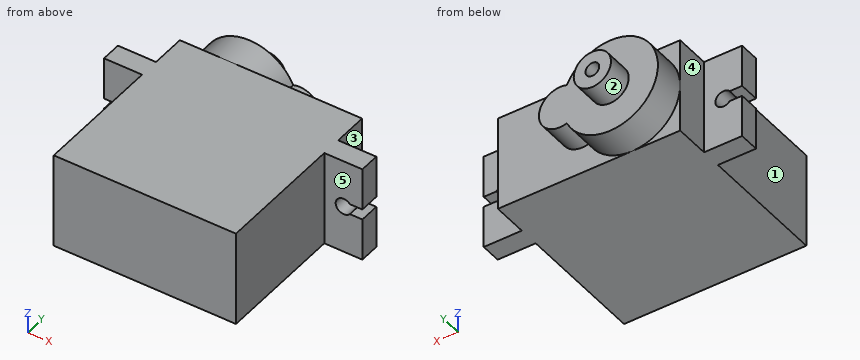
```python
from build123d import *

# Parameters (mm, degrees)
ESBO_O1_W                  = 22.5
ESBO_O1_H                  = 11.8
RESSALTO_EXTRUS_O1_DEPTH   = 22.7
ESBO_O2_W                  = 11.8
ESBO_O2_H                  = 2.5
RESSALTO_EXTRUS_O2_DEPTH   = 4.7
RESSALTO_EXTRUS_O3_DEPTH   = 4.7
RESSALTO_EXTRUS_O4_DEPTH   = 4
ESBO_O5_R                  = 2.3
ESBO_O5_R_2                = 0.85
RESSALTO_EXTRUS_O5_DEPTH   = 3.2
CORTE_EXTRUS_O1_DEPTH      = 35.894698738
CORTE_EXTRUS_O1_DEPTH_BACK = 3.2
CORTE_EXTRUS_O2_DEPTH      = 35.894698738
CORTE_EXTRUS_O2_DEPTH_BACK = 3.2


with BuildPart() as part:
    # Esboço1 → Ressalto-extrusão1 (new body)
    with BuildSketch(Plane(origin=(0, 0, 0), x_dir=(1, 0, 0), z_dir=(0, 1, 0))):
        with Locations((11.25, 5.9)):
            Rectangle(ESBO_O1_W, ESBO_O1_H)
    extrude(amount=RESSALTO_EXTRUS_O1_DEPTH)

    # Esboço2 → Ressalto-extrusão2 (add)
    with BuildSketch(Plane.ZY):
        with Locations((-5.9, 17.15)):
            Rectangle(ESBO_O2_W, ESBO_O2_H)
    extrude(amount=RESSALTO_EXTRUS_O2_DEPTH)

    # Esboço3 → Ressalto-extrusão3 (add)
    with BuildSketch(Plane(origin=(22.5, 0, 0), x_dir=(0, 0, -1), z_dir=(1, 0, 0))):
        Polygon((5.9, 15.9), (11.8, 15.9), (11.8, 18.4), (0, 18.4), (0, 15.9), align=None)
    extrude(amount=RESSALTO_EXTRUS_O3_DEPTH)

    # Esboço4 → Ressalto-extrusão4 (add)
    with BuildSketch(Plane(origin=(0, 22.7, 0), x_dir=(1, 0, 0), z_dir=(0, 1, 0))):
        with BuildLine():
            ThreePointArc((11.244155686, 8.4), (0, 5.9), (11.244155686, 3.4))
            ThreePointArc((11.244155686, 3.4), (14.7, 5.9), (11.244155686, 8.4))
        make_face()
    extrude(amount=RESSALTO_EXTRUS_O4_DEPTH)

    # Esboço5 → Ressalto-extrusão5 (add)
    with BuildSketch(Plane(origin=(0, 26.7, 0), x_dir=(1, 0, 0), z_dir=(0, 1, 0))):
        with Locations(Location((5.9, 5.9, 0), (0, 0, 90))):
            Circle(ESBO_O5_R)
        with Locations(Location((5.9, 5.9, 0), (0, 0, 270))):
            Circle(ESBO_O5_R_2, mode=Mode.SUBTRACT)
    extrude(amount=RESSALTO_EXTRUS_O5_DEPTH)

    # Esboço6 → Corte-extrusão1 (cut, two sides: drawn at the far end of the back side and taken through both)
    with BuildSketch(Plane(origin=(0, 18.4, 0), x_dir=(1, 0, 0), z_dir=(0, 1, 0)).offset(-CORTE_EXTRUS_O1_DEPTH_BACK)):
        with BuildLine():
            Line((-3.159934208, 6.55), (-4.7, 6.55))
            Line((-4.7, 6.55), (-4.7, 5.25))
            Line((-4.7, 5.25), (-3.159934208, 5.25))
            ThreePointArc((-3.159934208, 5.25), (-1.4, 5.9), (-3.159934208, 6.55))
        make_face()
    extrude(amount=CORTE_EXTRUS_O1_DEPTH + CORTE_EXTRUS_O1_DEPTH_BACK, mode=Mode.SUBTRACT)

    # Esboço7 → Corte-extrusão2 (cut, two sides: drawn at the far end of the back side and taken through both)
    with BuildSketch(Plane(origin=(0, 18.4, 0), x_dir=(1, 0, 0), z_dir=(0, 1, 0)).offset(-CORTE_EXTRUS_O2_DEPTH_BACK)):
        with BuildLine():
            Line((25.659934208, 5.25), (27.2, 5.25))
            Line((27.2, 5.25), (27.2, 6.55))
            Line((27.2, 6.55), (25.659934208, 6.55))
            ThreePointArc((25.659934208, 6.55), (23.9, 5.9), (25.659934208, 5.25))
        make_face()
    extrude(amount=CORTE_EXTRUS_O2_DEPTH + CORTE_EXTRUS_O2_DEPTH_BACK, mode=Mode.SUBTRACT)


solid = part.part
```
Work out the finished part from the listing and answer in its coordinate system (mm). Face numbers are marked on the shaded views. A direction names the side the tool comes from. Coordinates: 2 decimals unless noted, no trailing zeros. Order: outer loops, then holes, each group sorted by start corner. A loop starts at its lowest first (then second) coordinate and runs counter-clockwise, first axis right, second up. Notation, with made-up numbers: M 69,-13 L 74,-13 A25 ccw 74,15 Z; hole C 47,-6.5 d11. An arc over 180 degrees is marked long. Use CSV: the item, a comma, the result in double quotes.
1) For the marked faces 1, 2, 3, 4 and 5, determine the directions among +Z, -Z, +X, -X, +Y, -Y from which every point of the face is accessible in a straight line to the end or side of a thin tool.
Worked out:
face 1,"+Z, -Z, -X, -Y"
face 2,"+Y"
face 3,"+Z, -Z, +X, +Y"
face 4,"+Z, -Z, -X, +Y"
face 5,"+Z, -Z, +X, -Y"
2) Section C-C on y = 13.5 is taken. Write down the section's boundary in (x, z), plus the area to 4 significant figures.
Worked out:
outline,"M 0,-11.8 L 22.5,-11.8 L 22.5,0 L 0,0 Z"
area,"265.5 mm^2"
3) Consider line 1 (Z direction, x = 24.9, y = 17.2); line 2 (X direction, y = 27.4, z = -5.9); line 3 (Y direction, x = 13.5, z = -8). Determine where each line is inside the solid, lowest interval first. Write a range as [from, to].
Worked out:
line 1,"z = [-11.8, -6.9], [-4.9, 0]"
line 2,"x = [3.6, 5.05], [6.75, 8.2]"
line 3,"y = [0, 26.7]"
4) Section A-A on x = -2.4 is taken. Write down the section's boundary in (y, z), plus the area to 3 significant figures.
Worked out:
outline,"M 15.9,-11.8 L 18.4,-11.8 L 18.4,-6.9 L 15.9,-6.9 Z; M 15.9,-4.9 L 18.4,-4.9 L 18.4,0 L 15.9,0 Z"
area,"24.5 mm^2"
5) Section B-B on z = -4.5 is taken. Write down the section's boundary in (x, y), plus the area to 3 significant figures.
Worked out:
outline,"M -4.7,15.9 L 0,15.9 L 0,0 L 22.5,0 L 22.5,15.9 L 27.2,15.9 L 27.2,18.4 L 22.5,18.4 L 22.5,22.7 L 14.3,22.7 L 14.3,26.7 L 7.72,26.7 L 7.72,29.9 L 4.08,29.9 L 4.08,26.7 L 0.17,26.7 L 0.17,22.7 L 0,22.7 L 0,18.4 L -4.7,18.4 Z"
area,"602 mm^2"
6) Section D-D on z = -9.25 is taken. Write down the section's boundary in (x, y).
Worked out:
outline,"M -4.7,15.9 L 0,15.9 L 0,0 L 22.5,0 L 22.5,15.9 L 27.2,15.9 L 27.2,18.4 L 22.5,18.4 L 22.5,22.7 L 10.76,22.7 L 10.76,26.7 L 1.04,26.7 L 1.04,22.7 L 0,22.7 L 0,18.4 L -4.7,18.4 Z"
7) Flat-ended cylindrical pins translate along their axes: pin 1 Ø3.5 at (x, z) = (13, -5) entering from +Y; pin 2 Ø4.5 at (y, z) = (21.5, -6.5) entering from -X; pin 3 Ø3.5 at (y, z) = (21, -3) entering from +X; pin 4 Ø1.8 at (x, z) = (-2.4, -5.9) entering from +Y. Find the tip coordinate at first contact, or state that the pin passes through.
Worked out:
pin 1,"stops at y = 26.7"
pin 2,"stops at x = 0"
pin 3,"stops at x = 22.5"
pin 4,"passes through"
